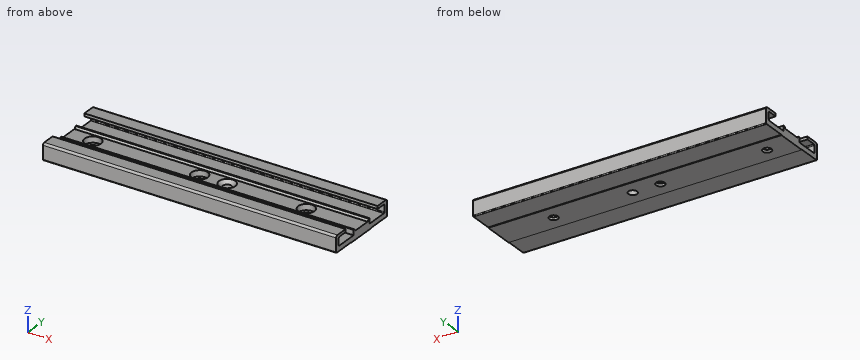
from build123d import *

# Parameters (mm, degrees)
BOSS_EXTRUDE1_DEPTH                                 = 152.4
CBORE_FOR_0_BINDING_HEAD_MACHINE_SCREW1_D           = 4.499991
CBORE_FOR_0_BINDING_HEAD_MACHINE_SCREW1_CBORE_D     = 8.5000084
CBORE_FOR_0_BINDING_HEAD_MACHINE_SCREW1_CBORE_DEPTH = 3.099999896
CSK_FOR_0_FLAT_HEAD_MACHINE_SCREW_100_D             = 4.499991
CSK_FOR_0_FLAT_HEAD_MACHINE_SCREW_100_CSINK_D       = 8.5000084
CSK_FOR_0_FLAT_HEAD_MACHINE_SCREW_100_CSINK_ANGLE   = 100


with BuildPart() as part:
    # Sketch1 → Boss-Extrude1 (new body)
    with BuildSketch(Plane(origin=(0, 0, 0), x_dir=(0, 0, -1), z_dir=(1, 0, 0))):
        with BuildLine():
            Line((-8.7, -12.5), (-8.7, -19))
            ThreePointArc((-8.7, -19), (-8.407106781, -19.707106781), (-7.7, -20))
            Line((-7.7, -20), (-0.7, -20))
            ThreePointArc((-0.7, -20), (-0.346446609, -19.853553391), (-0.2, -19.5))
            Line((-0.2, -19.5), (-0.2, -8))
            Line((-0.2, -8), (0, -8))
            Line((0, -8), (0, 8))
            Line((0, 8), (-0.2, 8))
            Line((-0.2, 8), (-0.2, 19.5))
            ThreePointArc((-0.2, 19.5), (-0.346446609, 19.853553391), (-0.7, 20))
            Line((-0.7, 20), (-7.7, 20))
            ThreePointArc((-7.7, 20), (-8.407106781, 19.707106781), (-8.7, 19))
            Line((-8.7, 19), (-8.7, 12.5))
            Line((-8.7, 12.5), (-7.2, 12.5))
            Line((-7.2, 12.5), (-7.2, 17.5))
            ThreePointArc((-7.2, 17.5), (-7.053553391, 17.853553391), (-6.7, 18))
            Line((-6.7, 18), (-3.3, 18))
            ThreePointArc((-3.3, 18), (-2.946446609, 17.853553391), (-2.8, 17.5))
            Line((-2.8, 17.5), (-2.8, 6.3))
            Line((-2.8, 6.3), (-5.5, 6.3))
            Line((-5.5, 6.3), (-5.5, 5.75))
            Line((-5.5, 5.75), (-4.5, 4.75))
            Line((-4.5, 4.75), (-4.5, -4.75))
            Line((-4.5, -4.75), (-5.5, -5.75))
            Line((-5.5, -5.75), (-5.5, -6.3))
            Line((-5.5, -6.3), (-2.8, -6.3))
            Line((-2.8, -6.3), (-2.8, -17.5))
            ThreePointArc((-2.8, -17.5), (-2.946446609, -17.853553391), (-3.3, -18))
            Line((-3.3, -18), (-6.7, -18))
            ThreePointArc((-6.7, -18), (-7.053553391, -17.853553391), (-7.2, -17.5))
            Line((-7.2, -17.5), (-7.2, -12.5))
            Line((-7.2, -12.5), (-8.7, -12.5))
        make_face()
    extrude(amount=BOSS_EXTRUDE1_DEPTH)

    # CBORE for #0 Binding Head Machine Screw1 (through all)
    with Locations(Plane.XY.offset(4.5)):
        with Locations((12.7, 0), (68.2, 0), (123.7, 0), (179.2, 0), (234.7, 0), (290.2, 0), (345.7, 0)):
            CounterBoreHole(CBORE_FOR_0_BINDING_HEAD_MACHINE_SCREW1_D / 2, CBORE_FOR_0_BINDING_HEAD_MACHINE_SCREW1_CBORE_D / 2, CBORE_FOR_0_BINDING_HEAD_MACHINE_SCREW1_CBORE_DEPTH)

    # CSK for #0 Flat Head Machine Screw (100)1 (through all)
    with Locations(Plane.XY.offset(4.5)):
        with Locations((82.55, 0)):
            CounterSinkHole(CSK_FOR_0_FLAT_HEAD_MACHINE_SCREW_100_D / 2, CSK_FOR_0_FLAT_HEAD_MACHINE_SCREW_100_CSINK_D / 2, counter_sink_angle=CSK_FOR_0_FLAT_HEAD_MACHINE_SCREW_100_CSINK_ANGLE)


solid = part.part
For this review, take the finished solid that the model builds, in its own axes (mm). Coordinates: 2 decimals unless noted, no trailing zeros. Order: outer loops, then holes, each group sorted by start corner. A loop starts at its lowest first (then second) coordinate and runs counter-clockwise, first axis right, second up. Notation, with made-up numbers: (36, 64.25) - (83, 64.25) arc R20 cw to (83, 72.25) - close; hole circle Ø8 at (0.5, -8.75). An arc over 180 degrees is marked (long way). Answer as CSV lines item,"result". Start each with the question number.
1) Add section B-B (y = 15.5). State the section outline as (x, z) points.
2) To check wall thickness, follow line 1 along Y through (x, z) = (54.5, 4); line 2 along Y through (x, z) = (110, 4.75); line 3 along Y through (x, z) = (37, 7.25). State the ranges of each line that lie inside material, in increasing order. Write a range as [from, to].
3) Add section A-A (y = 0). Count the separate pieces of the cut face and the enclosed holes in it, then the cut area to 3 significant figures.
4) Insertion check: P1, Ø11, axis at x = 12.7, y = 0, coming from the +Z side; P2, Ø1.5, axis at x = 109, y = 7.5, coming from the +Z side; P3, Ø1.5, axis at x = 42, y = 15.5, coming from the -Z side; P4, Ø1, axis at y = 7.5, z = 4.5, coming from the -X side. Each pin has a flat end and moves straight along its axis. Give the tip position at first contact, or say it passes through.
Result:
1,outline,"(0, 0.2) - (152.4, 0.2) - (152.4, 2.8) - (0, 2.8) - close; (0, 7.2) - (152.4, 7.2) - (152.4, 8.7) - (0, 8.7) - close"
2,line 1,"[-20, -18], [-6.3, 6.3], [18, 20]"
2,line 2,"[-20, -18], [-6.3, -5], [5, 6.3], [18, 20]"
2,line 3,"[-20, -12.5], [12.5, 20]"
3,separate pieces,"5"
3,enclosed holes,"0"
3,area,"564 mm^2"
4,P1,"z = 5.25"
4,P2,"z = 2.8"
4,P3,"z = 0.2"
4,P4,"through"
